Check sheet for the drawn part. Datum: minimum x, y, z corner. Units: mm. Coordinates: 2 decimals unless noted, no trailing zeros. Order: outer loops, then holes, each group sorted by start corner. A loop starts at its lowest first (then second) coordinate and runs counter-clockwise, first axis right, second up. Notation, with made-up numbers: M 30,6 L 71,6 A16 ccw 71,34 Z; hole C 19.5,55.25 d11. An arc over 180 degrees is marked long. Use one line per item in the form item = value. Start each with the question number.
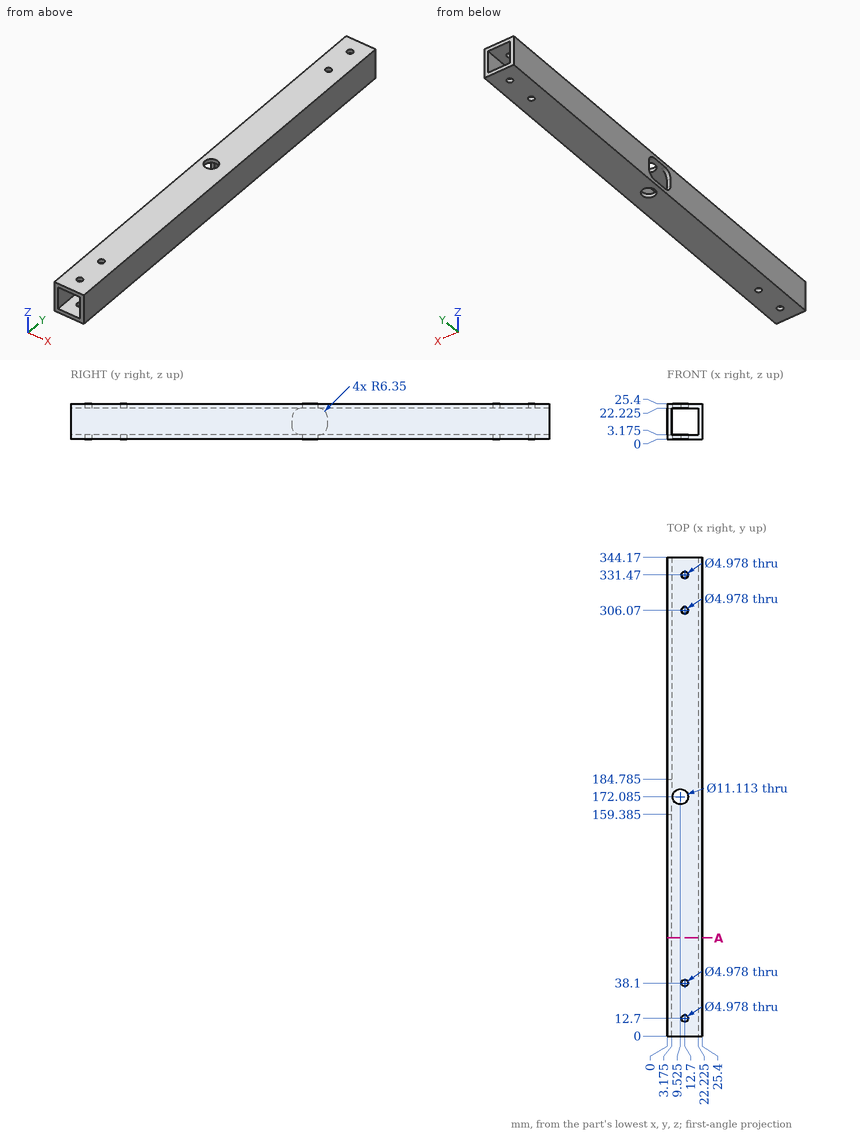
1. Depth check by flat-ended pin: P1, Ø10, axis at x = 9.525, y = 172.085, coming from the -Z side. Enter the tip coordinate at first touch or a pass-through.
2. Material ranges on line 1 along X through (y, z) = (66.5, 5.5) (1 decimal); line 2 along Y through (x, z) = (12.7, 2) (1 decimal), recorded low to high.
3. Cross-section at A-A on y = 70.5. Enter the section's corners in (x, z) (1 decimal).
Final values:
q1.P1 = through
q2.line_1 = 0 to 3.2, 22.2 to 25.4
q2.line_2 = 0 to 10.2, 15.2 to 35.6, 40.6 to 167.5, 176.6 to 303.6, 308.6 to 329, 334 to 344.2
q3.outline = M 0,0 L 25.4,0 L 25.4,25.4 L 0,25.4 Z; hole M 3.2,3.2 L 22.2,3.2 L 22.2,22.2 L 3.2,22.2 Z
